from build123d import *

# Parameters (mm, degrees)
SKIZZE1_W                       = 86
SKIZZE1_H                       = 50
AUFSATZ_LINEAR_AUSTRAGEN1_DEPTH = 2
F_1_6_1_6_DIAMETER_HOLE1_D      = 1.6
M3X0_5_GEWINDEBOHRUNG1_D        = 2.5
M3X0_5_GEWINDEBOHRUNG1_DEPTH    = 8.5
M3X0_5_GEWINDEBOHRUNG1_TIP      = 0.751075774
SKIZZE6_W                       = 27.5
SKIZZE6_H                       = 34
SCHNITT_LINEAR_AUSTRAGEN1_DEPTH = 3
FILLET1_R                       = 3
CUT_EXTRUDE1_REACH              = 4
SKETCH1_W                       = 20
SKETCH1_H                       = 20
BOSS_EXTRUDE1_DEPTH             = 2
FILLET2_R                       = 3


with BuildPart() as part:
    # Skizze1 → Aufsatz-Linear austragen1 (new body)
    with BuildSketch(Plane(origin=(0, 0, 0), x_dir=(1, 0, 0), z_dir=(0, 1, 0))):
        Rectangle(SKIZZE1_W, SKIZZE1_H)
    extrude(amount=AUFSATZ_LINEAR_AUSTRAGEN1_DEPTH)

    # Ø1.6 (1.6) Diameter Hole1 (through all)
    with Locations(Plane(origin=(0, 2, 0), x_dir=(1, 0, 0), z_dir=(0, 1, 0))):
        with Locations((-39.45, 21.275), (-3, 21.275), (-3, -21.275)):
            f_1_6_1_6_diameter_hole1 = Hole(F_1_6_1_6_DIAMETER_HOLE1_D / 2)

    # Spiegeln1: Ø1.6 (1.6) Diameter Hole1 across plane
    add(f_1_6_1_6_diameter_hole1.mirror(Plane(origin=(0, 0, 0), x_dir=(0, 0, 1), z_dir=(1, 0, 0))), mode=Mode.SUBTRACT)

    # M3x0.5 Gewindebohrung1
    with Locations(Plane(origin=(0, 2, 0), x_dir=(1, 0, 0), z_dir=(0, 1, 0))):
        with Locations((0, 15), (0, -15)):
            Hole(M3X0_5_GEWINDEBOHRUNG1_D / 2, depth=M3X0_5_GEWINDEBOHRUNG1_DEPTH)
            with Locations((0, 0, -(M3X0_5_GEWINDEBOHRUNG1_DEPTH + M3X0_5_GEWINDEBOHRUNG1_TIP / 2))):  # 118° drill point
                Cone(0, M3X0_5_GEWINDEBOHRUNG1_D / 2, M3X0_5_GEWINDEBOHRUNG1_TIP, mode=Mode.SUBTRACT)

    # Skizze6 → Schnitt-Linear austragen1 (cut, through all)
    with BuildSketch(Plane(origin=(0, 0, 0), x_dir=(1, 0, 0), z_dir=(0, 1, 0))):
        with Locations((-21.25, 0)):
            Rectangle(SKIZZE6_W, SKIZZE6_H)
        with Locations((21.25, 0)):
            Rectangle(SKIZZE6_W, SKIZZE6_H)
    extrude(amount=SCHNITT_LINEAR_AUSTRAGEN1_DEPTH, mode=Mode.SUBTRACT)

    # Fillet1
    fillet1_edges = [part.edges().sort_by_distance(p)[0] for p in [
        (-43, 1, -25),
        (43, 1, -25),
        (43, 1, 25),
        (-43, 1, 25),
    ]]
    fillet(fillet1_edges, radius=FILLET1_R)

    # Sketch1 → Cut-Extrude1 (cut, up to next)
    with BuildSketch(Plane(origin=(0, 2, 0), x_dir=(1, 0, 0), z_dir=(0, 1, 0)), mode=Mode.PRIVATE) as cut_extrude1_sk1:
        with Locations((-33, -15)):
            Rectangle(SKETCH1_W, SKETCH1_H)
    cut_extrude1_tool1 = extrude(cut_extrude1_sk1.sketch, amount=-CUT_EXTRUDE1_REACH, mode=Mode.PRIVATE) & part.part
    add(cut_extrude1_tool1.solids().sort_by_distance((-33, 2, 15))[0], mode=Mode.SUBTRACT)

    # Sketch2 → Boss-Extrude1 (add)
    with BuildSketch(Plane(origin=(0, 2, 0), x_dir=(1, 0, 0), z_dir=(0, 1, 0))):
        Polygon((-43, -5), (-23, -25), (-23, -17), (-19.686291501, -17), (-35, -1.686291501), (-35, -5), align=None)
    extrude(amount=-BOSS_EXTRUDE1_DEPTH)

    # Fillet2
    fillet2_edges = [part.edges().sort_by_distance(p)[0] for p in [
        (-43, 1, 5),
        (-23, 1, 25),
    ]]
    fillet(fillet2_edges, radius=FILLET2_R)


solid = part.part
CAD build for the part. Positions are in the model's coordinates, mm. A direction names the side the tool comes from. Coordinates: 2 decimals unless noted, no trailing zeros. Write each loop counter-clockwise with the first axis right and the second up, starting at its lowest first coordinate (ties: lowest second). Pieces come first, ordered by that corner, then holes. Notation, with made-up numbers: (45.5, 58) - (86.5, 58) arc R20 ccw to (86.5, 71) - close; hole circle Ø4 at (-8.75, 63). An arc over 180 degrees is marked (long way). Use a Markdown table: item, result. Add a question column.
Item 1: Band-saw the part on A-A, the plane z = -11. Give the cut face in (x, y).
Item 2: Flat gauge pins, fed straight in: pin 1 (1 mm diameter, centred on x = -3, z = 21.275, fed in from +Y); pin 2 (0.6 mm diameter, centred on y = 0.5, z = 5, fed in from -X). Where does each tip first touch, or does it go through?
Item 3: Band-saw the part on D-D, the plane z = 15. Give the cut face in (x, y).
Item 4: Band-saw the part on B-B, the plane x = 29.5. Give the cut face in (y, z).
Item 5: 3-axis set-ups, long thin cutter, end or side, ignore diameter. For faces 4 (the face through (21, 1, -17)), 5 (the face through (42.1, 1.01, 24.14)): which of +Z, -Z, +X, -X, +Y, -Y reach the whole face in a straight line?
Item 6: Drill centre lines: L1, parallel to X at y = 1.2, z = -1; L2, parallel to Z at x = 3, y = 1.6 (3 decimals); L3, parallel to X at y = 1.4, z = -15. Where is each one in solid material? Low to high. Write a range as from..to.
Item 7: Mould opens along X. For faces 1 (the face through (7.5, 1, 0)), 2 (the face through (-1, 2, -6)), 3 (the face through (43, 1, 0)) say: pulls with the +X half, pulls with the -X half, needs draft (parallel to the pull), parting line crosses it, or undercut.
Item 8: Band-saw the part on C-C, the plane x = -3. Give the cut face in (y, z) (3 decimals), and give its area (3 significant figures).
Numbers:
| question | item | result |
|---|---|---|
| 1 | outline | (-43, 0) - (-35, 0) - (-35, 2) - (-43, 2) - close; (-7.5, 0) - (7.5, 0) - (7.5, 2) - (-7.5, 2) - close; (35, 0) - (43, 0) - (43, 2) - (35, 2) - close |
| 2 | pin 1 | through |
| 2 | pin 2 | x = -42.85 |
| 3 | outline | (-33, 0) - (-21.69, 0) - (-21.69, 2) - (-33, 2) - close; (-7.5, 0) - (-1.25, 0) - (-1.25, 2) - (-7.5, 2) - close; (1.25, 0) - (7.5, 0) - (7.5, 2) - (1.25, 2) - close; (35, 0) - (43, 0) - (43, 2) - (35, 2) - close |
| 4 | outline | (0, -25) - (2, -25) - (2, -17) - (0, -17) - close; (0, 17) - (2, 17) - (2, 25) - (0, 25) - close |
| 5 | face 4 | +Y, -Y |
| 5 | face 5 | +Z, +X, +Y, -Y |
| 6 | L1 | -43..-35, -7.5..7.5, 35..43 |
| 6 | L2 | -25..-22.075, -20.475..20.475, 22.075..25 |
| 6 | L3 | -43..-35, -7.5..-1.25, 1.25..7.5, 35..43 |
| 7 | face 1 | undercut |
| 7 | face 2 | needs draft |
| 7 | face 3 | pulls with the +X half |
| 8 | outline | (0, -25) - (2, -25) - (2, -22.075) - (0, -22.075) - close; (0, -20.475) - (2, -20.475) - (2, 20.475) - (0, 20.475) - close; (0, 22.075) - (2, 22.075) - (2, 25) - (0, 25) - close |
| 8 | area | 93.6 mm2 |
